Model file for the job. Use its own axes, mm. Coordinates: 2 decimals unless noted, no trailing zeros. Write each loop counter-clockwise with the first axis right and the second up, starting at its lowest first coordinate (ties: lowest second). Pieces come first, ordered by that corner, then holes. Notation, with made-up numbers: (82.25, -38.5) -> (96.25, -38.5) arc R23 cw to (96.25, -21.5) -> close; hole circle Ø1 at (69, 26). An arc over 180 degrees is marked (long way). Answer as a JSON object with one key per item and string values. Group by question number.
from build123d import *

# Parameters (mm, degrees)
F0_W     = 101.6
F0_H     = 50.8
F1_DEPTH = 50.8
F3_DEPTH = 50.801
F4_R     = 6.35
F5_DEPTH = 101.601


with BuildPart() as f1:
    # F0 (on Top) → F1 (new body)
    with BuildSketch(Plane.XY):
        with Locations((50.8, 25.4)):
            Rectangle(F0_W, F0_H)
    extrude(amount=F1_DEPTH)

    # F2 (on face) → F3 (cut, through all)
    with BuildSketch(Plane.XY.offset(50.8)):
        with BuildLine():
            Line((101.6, 12.7), (101.6, 38.1))
            ThreePointArc((101.6, 38.1), (88.9, 25.4), (101.6, 12.7))
        make_face()
    extrude(amount=-F3_DEPTH, mode=Mode.SUBTRACT)

    # F4 (on face) → F5 (cut, through all)
    with BuildSketch(Plane(origin=(0, 0, 0), x_dir=(0, -1, 0), z_dir=(-1, 0, 0))):
        with Locations((-25.4, 12.7)):
            Circle(F4_R)
    extrude(amount=-F5_DEPTH, mode=Mode.SUBTRACT)


solid = f1.part
(1) Cut at D-D on z = 45. List the corners of the cut face in (x, y).
(2) Pull direction Y, two halves, no side cores. Call faces 1 (the face through (50, 0, 25)), 2 (the face through (50, 50.8, 25)), 3 (the face through (88.903, 25.679, 25.756)), 4 (the face through (44.667, 21.986, 18.054)): released by +Y, released by -Y, zero draft, split by the parting line, or undercut.
(3) Cut at B-B on y = 25.4. List the corners of the cut face in (x, z).
(4) Cut at A-A on z = 12.7. List the corners of the cut face in (x, y), plus the area to 3 significant figures.
(5) Cut at C-C on x = 41. List the corners of the cut face in (y, z), plus the area to 3 significant figures.
(6) Pin check, flat tip, straight feed: pin 1 (2 mm diameter, centred on y = 17, z = 37.5, fed in from +X). Stop position of the tip, or through.
(7) Wall check: probe 1 along Z at (x, y) = (48.5, 25.4); probe 2 along Y at (x, z) = (27, 12.7); probe 3 along X at (y, z) = (27, 32). Give the ranges that are in metal, low to high.
Results found:
{
 "1": {"outline": "(0, 0) -> (101.6, 0) -> (101.6, 12.7) arc R12.7 cw to (101.6, 38.1) -> (101.6, 50.8) -> (0, 50.8) -> close"},
 "2": {"face 1": "released by -Y", "face 2": "released by +Y", "face 3": "undercut", "face 4": "undercut"},
 "3": {"outline": "(0, 0) -> (88.9, 0) -> (88.9, 6.35) -> (0, 6.35) -> close; (0, 19.05) -> (88.9, 19.05) -> (88.9, 50.8) -> (0, 50.8) -> close"},
 "4": {"outline": "(0, 0) -> (101.6, 0) -> (101.6, 12.7) arc R12.7 cw to (90.6, 19.05) -> (0, 19.05) -> close; (0, 31.75) -> (90.6, 31.75) arc R12.7 cw to (101.6, 38.1) -> (101.6, 50.8) -> (0, 50.8) -> close", "area": "3,770 mm²"},
 "5": {"outline": "(0, 0) -> (50.8, 0) -> (50.8, 50.8) -> (0, 50.8) -> close; hole circle Ø12.7 at (25.4, 12.7)", "area": "2,450 mm²"},
 "6": {"pin 1": "stops at x = 93.06"},
 "7": {"probe 1": "z = 0 to 6.35, 19.05 to 50.8", "probe 2": "y = 0 to 19.05, 31.75 to 50.8", "probe 3": "x = 0 to 89"}
}
